```python
from build123d import *

# Parameters (mm, degrees)
SKETCH1_R               = 12.5
BOSS_EXTRUDE1_DEPTH     = 50
SKETCH6_R               = 12.5
SKETCH6_R_2             = 6.85
CUT_EXTRUDE4_DEPTH      = 3
SKETCH7_R               = 3.955
BOSS_EXTRUDE3_DEPTH     = 45
SKETCH8_R               = 2.15
CUT_EXTRUDE5_DEPTH      = 13.5
CUT_EXTRUDE5_DEPTH_BACK = 13.5
SKETCH9_R               = 3.97
SKETCH9_R_2             = 3.8
CUT_EXTRUDE6_DEPTH      = 0.9
SKETCH10_R              = 4
CUT_EXTRUDE7_DEPTH      = 20
CHAMFER2_SIZE           = 2.5
CHAMFER3_SIZE           = 2.5
CHAMFER4_SIZE           = 1
SKETCH2_R               = 8.963089754
BOSS_EXTRUDE2_DEPTH     = 35
SKETCH12_R              = 9.5
SKETCH12_R_2            = 4.5
BOSS_EXTRUDE4_DEPTH     = 9
SKETCH11_W              = 8.2
SKETCH11_H              = 13.7
CUT_EXTRUDE8_DEPTH      = 13.5
CUT_EXTRUDE8_DEPTH_BACK = 13.5
SKETCH13_R              = 4.5
CUT_EXTRUDE9_DEPTH      = 17
CHAMFER5_SIZE           = 0.5


with BuildPart() as part:
    # Sketch1 → Boss-Extrude1 (new body)
    with BuildSketch(Plane(origin=(0, 0, 0), x_dir=(0, 0, -1), z_dir=(1, 0, 0))):
        Circle(SKETCH1_R)
    extrude(amount=-BOSS_EXTRUDE1_DEPTH)

    # Sketch6 → Cut-Extrude4 (cut)
    with BuildSketch(Plane(origin=(0, 0, 0), x_dir=(0, 0, -1), z_dir=(1, 0, 0))):
        Circle(SKETCH6_R)
        Circle(SKETCH6_R_2, mode=Mode.SUBTRACT)
    extrude(amount=-CUT_EXTRUDE4_DEPTH, mode=Mode.SUBTRACT)

    # Sketch7 → Boss-Extrude3 (add)
    with BuildSketch(Plane(origin=(0, 0, 0), x_dir=(0, 0, -1), z_dir=(1, 0, 0))):
        Circle(SKETCH7_R)
    extrude(amount=BOSS_EXTRUDE3_DEPTH)

    # Sketch8 → Cut-Extrude5 (cut, two sides)
    with BuildSketch(Plane.XY) as cut_extrude5_sk:
        with Locations((33.94, 0)):
            Circle(SKETCH8_R)
    extrude(amount=CUT_EXTRUDE5_DEPTH, mode=Mode.SUBTRACT)
    extrude(cut_extrude5_sk.sketch, amount=-CUT_EXTRUDE5_DEPTH_BACK, mode=Mode.SUBTRACT)

    # Sketch9 → Cut-Extrude6 (cut)
    with BuildSketch(Plane(origin=(40.2, 0, 0), x_dir=(0, 0, -1), z_dir=(1, 0, 0))):
        Circle(SKETCH9_R)
        Circle(SKETCH9_R_2, mode=Mode.SUBTRACT)
    extrude(amount=CUT_EXTRUDE6_DEPTH, mode=Mode.SUBTRACT)

    # Sketch10 → Cut-Extrude7 (cut)
    with BuildSketch(Plane.ZY.offset(50)):
        Circle(SKETCH10_R)
    extrude(amount=-CUT_EXTRUDE7_DEPTH, mode=Mode.SUBTRACT)

    # Chamfer2
    chamfer2_edges = [part.edges().sort_by_distance(p)[0] for p in [
        (-50, 0, 12.5),
    ]]
    chamfer(chamfer2_edges, length=CHAMFER2_SIZE)

    # Chamfer3
    chamfer3_edges = [part.edges().sort_by_distance(p)[0] for p in [
        (-3, 0, 12.5),
    ]]
    chamfer(chamfer3_edges, length=CHAMFER3_SIZE)

    # Chamfer4
    chamfer4_edges = [part.edges().sort_by_distance(p)[0] for p in [
        (45, 0, 3.955),
    ]]
    chamfer(chamfer4_edges, length=CHAMFER4_SIZE)

    # Sketch2 → Boss-Extrude2 (add)
    with BuildSketch(Plane.ZY.offset(50)):
        Circle(SKETCH2_R)
    extrude(amount=-BOSS_EXTRUDE2_DEPTH)

    # Sketch12 → Boss-Extrude4 (add)
    with BuildSketch(Plane.ZY.offset(50)):
        Circle(SKETCH12_R)
        Circle(SKETCH12_R_2, mode=Mode.SUBTRACT)
    extrude(amount=-BOSS_EXTRUDE4_DEPTH)

    # Sketch11 → Cut-Extrude8 (cut, two sides)
    with BuildSketch(Plane(origin=(0, 0, 0), x_dir=(1, 0, 0), z_dir=(0, 1, 0))) as cut_extrude8_sk:
        with Locations((-37.5, 0)):
            Rectangle(SKETCH11_W, SKETCH11_H)
    extrude(amount=CUT_EXTRUDE8_DEPTH, mode=Mode.SUBTRACT)
    extrude(cut_extrude8_sk.sketch, amount=-CUT_EXTRUDE8_DEPTH_BACK, mode=Mode.SUBTRACT)

    # Sketch13 → Cut-Extrude9 (cut)
    with BuildSketch(Plane.ZY.offset(50)):
        Circle(SKETCH13_R)
    extrude(amount=-CUT_EXTRUDE9_DEPTH, mode=Mode.SUBTRACT)

    # Chamfer5
    chamfer5_edges = [part.edges().sort_by_distance(p)[0] for p in [
        (0, 0, 3.955),
    ]]
    chamfer(chamfer5_edges, length=CHAMFER5_SIZE)


solid = part.part
```
Read the model definition and answer for the solid it produces. Units are mm, in the model's axes. A direction names the side the tool comes from. Give positions to 0.01 mm unless a question says otherwise; leave off trailing zeros. Write each loop counter-clockwise with the first axis right and the second up, starting at its lowest first coordinate (ties: lowest second). Pieces come first, ordered by that corner, then holes. Notation, with made-up numbers: (34, 28) -> (85, 28) arc R37 ccw to (85, 66) -> close; hole circle Ø1 at (74.25, 31.25). An arc over 180 degrees is marked (long way). Answer in a Markdown table with one row per item.
1) A tool of negligible diameter and unlimited length cuts with its end or side. For faces 1 (the cylindrical face through (-1.48, 4.63, 5.05)), 2 (the flat face through (-33, 0, 0)), 3 (the flat face through (-41.6, 0, 5)), from which of +Z, -Z, +X, -X, +Y, -Y can it reach the whole face along a straight path? Write none if from no direction.
Results list:
| item | result |
|---|---|
| face 1 | +X |
| face 2 | -X |
| face 3 | +Y, -Y |
2) Determine the mould class of faces 4 (the cylindrical face through (31.79, 0.09, 0.06)), 5 (the cylindrical face through (-45.86, 4.46, -0.59)), 6 (the flat face through (-38, 0, 6.85)), 7 (the cylindrical face through (42.53, -3.86, 0.86)) for opening direction Y: released by +Y, released by -Y, zero draft, split by the parting line, or undercut.
Results list:
| item | result |
|---|---|
| face 4 | undercut |
| face 5 | undercut |
| face 6 | zero draft |
| face 7 | split by the parting line |
3) Straight lines are drawn through the part: line 1 (Z direction, x = -35, y = -0.5); line 2 (X direction, y = 0, z = -0.25); line 3 (X direction, y = 5.5, z = 1.25). For each, find the intervals that lie inside material, in ascending order. Write a range as [from, to].
Results list:
| item | result |
|---|---|
| line 1 | [-12.49, -6.85], [6.85, 12.49] |
| line 2 | [-33, 31.79], [36.09, 45] |
| line 3 | [-50, -41.6], [-33.4, 0] |
4) Section D-D on x = 33.94 is taken. Give the vertices of the cut face in (y, z) (3 decimals).
Results list:
| item | result |
|---|---|
| outline | (-2.15, -3.32) -> (-2.15, 3.32) arc R3.955 ccw to start; (2.15, -3.32) arc R3.955 ccw to (2.15, 3.32) -> close |
5) Section C-C on x = 3.5 is taken. Give the vertices of the cut face in (y, z) (3 decimals).
Results list:
| item | result |
|---|---|
| outline | circle Ø7.91 at (0, 0) |
6) Section B-B on x = -36 is taken. Give the vertices of the cut face in (y, z), plus the area to 3 significant figures.
Results list:
| item | result |
|---|---|
| outline | (-10.46, -6.85) arc R12.5 ccw to (10.46, -6.85) -> close; (-10.46, 6.85) -> (10.46, 6.85) arc R12.5 ccw to start |
| area | 166 mm^2 |
7) Each of these flat-tipped pins is pushed along its axis until it touches: pin 1 Ø6.5 at (y, z) = (0.5, -0.5) entering from -X; pin 2 Ø5 at (x, z) = (14, 7) entering from +Y; pin 3 Ø6 at (y, z) = (0.5, 1.5) entering from -X; pin 4 Ø3 at (x, y) = (34.5, -2.5) entering from -Z. Where does it stop, or does it pass through?
Results list:
| item | result |
|---|---|
| pin 1 | x = -33 |
| pin 2 | through |
| pin 3 | x = -50 |
| pin 4 | z = -3.69 |
8) Section A-A on z = 0 is taken. Count the separate pieces of the cut face and the enclosed holes in it, plus the area to 3 significant figures.
Results list:
| item | result |
|---|---|
| separate pieces | 3 |
| enclosed holes | 1 |
| area | 1,260 mm^2 |
